Could you check a few things on this model? Use its own coordinates, in mm. Coordinates: 2 decimals unless noted, no trailing zeros. Loops run counter-clockwise (first coordinate to the right, second up) from the corner with the lowest first, then second, coordinate; pieces in that order, holes last. Notation, with made-up numbers: (34.25, 78.25) - (62.25, 78.25) arc R16 cw to (62.25, 103.25) - close; hole circle Ø8 at (-33.5, -11). An arc over 180 degrees is marked (long way). One line per item, written item: value. Start each with the question number.
(1) If I drill on line 1 along X through (y, z) = (178.5, 2.2) (3 decimals); line 2 along Y through (x, z) = (76, 1.4); line 3 along Y through (x, z) = (109, 2.4), over which ranges is the centre line in solid material (lowest first)? Write a range as from..to.
(2) If we section it at B-B on y = 230: Write out the boundary of the cut face in (x, z) (3 decimals), then the cut area to 3 significant figures.
(3) If we section it at C-C on x = 91: Write out the boundary of the cut face in (y, z) (3 decimals), then the cut area to 3 significant figures.
(4) If we section it at A-A on z = 2.65: Write out the boundary of the cut face in (x, y) (3 decimals), then the cut area to 3 significant figures.
(5) I'm going to push a flat-ended pin straight in: P1, Ø1, axis at x = 41.5, z = 1, coming from the +Y side. Where does the tip first touch, or does it pass through?
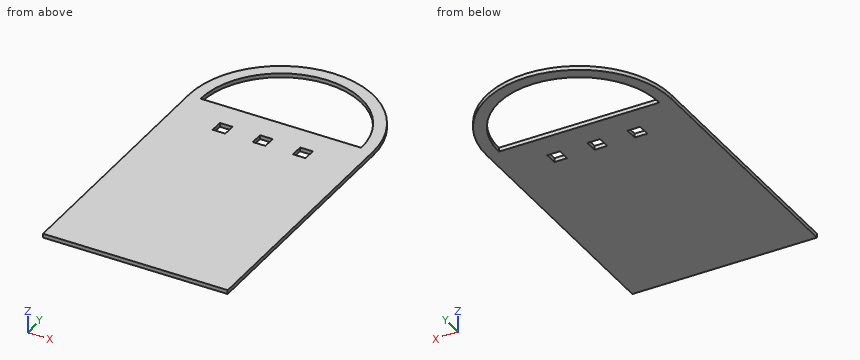
```python
from build123d import *

# Parameters (mm, degrees)
SKETCH2_W           = 10
SKETCH2_H           = 10
BOSS_EXTRUDE5_DEPTH = 3.175


with BuildPart() as part:
    # Sketch2 → Boss-Extrude5 (new body)
    with BuildSketch(Plane.XY):
        with BuildLine():
            Line((0, 0), (146.05, 0))
            Line((146.05, 0), (146.05, 203.2))
            ThreePointArc((146.05, 203.2), (73.025, 276.225), (0, 203.2))
            Line((0, 203.2), (0, 0))
        make_face()
        with BuildLine():
            Line((9.525, 203.2), (136.525, 203.2))
            ThreePointArc((136.525, 203.2), (73.025, 266.7), (9.525, 203.2))
        make_face(mode=Mode.SUBTRACT)
        with Locations((41.275, 177.8)):
            Rectangle(SKETCH2_W, SKETCH2_H, mode=Mode.SUBTRACT)
        with Locations((73.025, 177.8)):
            Rectangle(SKETCH2_W, SKETCH2_H, mode=Mode.SUBTRACT)
        with Locations((104.775, 177.8)):
            Rectangle(SKETCH2_W, SKETCH2_H, mode=Mode.SUBTRACT)
    extrude(amount=BOSS_EXTRUDE5_DEPTH)


solid = part.part
```
Values:
1. line 1: x = 0..36.275, 46.275..68.025, 78.025..99.775, 109.775..146.05
1. line 2: y = 0..172.8, 182.8..203.2, 266.63..276.16
1. line 3: y = 0..172.8, 182.8..203.2, 255.53..266.75
2. outline: (5.096, 0) - (15.458, 0) - (15.458, 3.175) - (5.096, 3.175) - close; (130.592, 0) - (140.954, 0) - (140.954, 3.175) - (130.592, 3.175) - close
2. area: 65.8 mm2
3. outline: (0, 0) - (203.2, 0) - (203.2, 3.175) - (0, 3.175) - close; (264.103, 0) - (273.978, 0) - (273.978, 3.175) - (264.103, 3.175) - close
3. area: 677 mm2
4. outline: (0, 0) - (146.05, 0) - (146.05, 203.2) arc R73.025 ccw to (0, 203.2) - close; hole (9.525, 203.2) - (136.525, 203.2) arc R63.5 ccw to start; hole (36.275, 172.8) - (46.275, 172.8) - (46.275, 182.8) - (36.275, 182.8) - close; hole (68.025, 172.8) - (78.025, 172.8) - (78.025, 182.8) - (68.025, 182.8) - close; hole (99.775, 172.8) - (109.775, 172.8) - (109.775, 182.8) - (99.775, 182.8) - close
4. area: 31,400 mm2
5. P1: stops at y = 269.31
